Design review of the part built by this model. Coordinates are the model's own, in mm. A direction names the side the tool comes from. Coordinates: 2 decimals unless noted, no trailing zeros. Order: outer loops, then holes, each group sorted by start corner. A loop starts at its lowest first (then second) coordinate and runs counter-clockwise, first axis right, second up. Notation, with made-up numbers: M -33.5,36.5 L 5.5,36.5 A18 ccw 5.5,59.5 Z; hole C -24.5,23 d7. An arc over 180 degrees is marked long. Answer as a JSON object with one key per item and string values.
from build123d import *

# Parameters (mm, degrees)
F0_R     = 16
F0_R_2   = 13.5
F1_DEPTH = 15.5
F2_W     = 4
F2_H     = 19.090906
F3_DEPTH = 25
F4_W     = 2
F4_H     = 0.5
F4_W_2   = 0.5
F4_H_2   = 2
F5_DEPTH = 25


with BuildPart() as f1:
    # F0 (on Front) → F1 (new body)
    with BuildSketch(Plane.XZ):
        Circle(F0_R)
        Circle(F0_R_2, mode=Mode.SUBTRACT)
    extrude(amount=F1_DEPTH)

    # F2 (on Top) → F3 (cut)
    with BuildSketch(Plane.XY):
        with Locations((0, -8.067074)):
            Rectangle(F2_W, F2_H)
    extrude(amount=-F3_DEPTH, mode=Mode.SUBTRACT)

    # F4 (on Front) → F5 (cut, symmetric)
    with BuildSketch(Plane.XZ):
        with Locations((0, 13.665518)):
            Rectangle(F4_W, F4_H)
        Polygon((-5.251188, 12.925427), (-5.09668, 12.449899), (-3.194566, 13.067933), (-3.349075, 13.543461), align=None)
        Polygon((-8.988353, 10.670105), (-8.694461, 10.265597), (-7.076427, 11.441167), (-7.370319, 11.845676), align=None)
        Polygon((-11.845676, 7.370319), (-11.441167, 7.076427), (-10.265597, 8.694461), (-10.670105, 8.988353), align=None)
        Polygon((-13.543461, 3.349075), (-13.067933, 3.194566), (-12.449899, 5.09668), (-12.925427, 5.251188), align=None)
        with Locations((-13.665518, 0)):
            Rectangle(F4_W_2, F4_H_2)
        Polygon((-12.925427, -5.251188), (-12.449899, -5.09668), (-13.067933, -3.194566), (-13.543461, -3.349075), align=None)
        Polygon((-10.670105, -8.988353), (-10.265597, -8.694461), (-11.441167, -7.076427), (-11.845676, -7.370319), align=None)
        Polygon((-7.370319, -11.845676), (-7.076427, -11.441167), (-8.694461, -10.265597), (-8.988353, -10.670105), align=None)
        Polygon((-3.349075, -13.543461), (-3.194566, -13.067933), (-5.09668, -12.449899), (-5.251188, -12.925427), align=None)
        with Locations((0, -13.665518)):
            Rectangle(F4_W, F4_H)
        Polygon((5.251188, -12.925427), (5.09668, -12.449899), (3.194566, -13.067933), (3.349075, -13.543461), align=None)
        Polygon((8.988353, -10.670105), (8.694461, -10.265597), (7.076427, -11.441167), (7.370319, -11.845676), align=None)
        Polygon((11.845676, -7.370319), (11.441167, -7.076427), (10.265597, -8.694461), (10.670105, -8.988353), align=None)
        Polygon((13.543461, -3.349075), (13.067933, -3.194566), (12.449899, -5.09668), (12.925427, -5.251188), align=None)
        with Locations((13.665518, 0)):
            Rectangle(F4_W_2, F4_H_2)
        Polygon((12.925427, 5.251188), (12.449899, 5.09668), (13.067933, 3.194566), (13.543461, 3.349075), align=None)
        Polygon((10.670105, 8.988353), (10.265597, 8.694461), (11.441167, 7.076427), (11.845676, 7.370319), align=None)
        Polygon((7.370319, 11.845676), (7.076427, 11.441167), (8.694461, 10.265597), (8.988353, 10.670105), align=None)
        Polygon((3.349075, 13.543461), (3.194566, 13.067933), (5.09668, 12.449899), (5.251188, 12.925427), align=None)
    extrude(amount=F5_DEPTH, both=True, mode=Mode.SUBTRACT)


solid = f1.part
1) Add section A-A (z = 0). State the section outline as (x, y) points.
Taken from the geometry:
{"outline": "M -16,-15.5 L -13.92,-15.5 L -13.92,0 L -16,0 Z; M 13.92,-15.5 L 16,-15.5 L 16,0 L 13.92,0 Z"}
2) Add section C-C (x = 0). State the section outline as (y, z) points, and give its area (3 significant figures).
Taken from the geometry:
{"outline": "M -15.5,13.92 L 0,13.92 L 0,16 L -15.5,16 Z", "area": "32.3 mm2"}
3) Tool access review of faces 1 (the flat face through (-2, -8, -15)), 2 (the flat face through (-4.31, -7.64, -13.23)): name each direction out of +Z, -Z, +X, -X, +Y, -Y from which nothing blocks a thin tool from reaching the whole face with its end or side.
Taken from the geometry:
{"face 1": "-Z, +Y, -Y", "face 2": "+Y, -Y"}
4) To check wall thickness, follow L1, parallel to X at y = -7.25, z = 0; L2, parallel to X at y = -13, z = -14; L3, parallel to Z at x = 0.5, y = -2.25. State the ranges of each line that lie inside material, in increasing order.
Taken from the geometry:
{"L1": "x = -16 to -13.92, 13.92 to 16", "L2": "x = -7.75 to -2, 2 to 7.75", "L3": "z = 13.92 to 15.99"}
5) Add section B-B (x = -6). State the section outline as (y, z) points.
Taken from the geometry:
{"outline": "M -15.5,-14.83 L 0,-14.83 L 0,-12.09 L -15.5,-12.09 Z; M -15.5,12.09 L 0,12.09 L 0,14.83 L -15.5,14.83 Z"}
6) Insertion check: pin 1 Ø6 at (x, y) = (0, -9) entering from -Z; pin 2 Ø4 at (y, z) = (-5, -2) entering from -X; pin 3 Ø4 at (y, z) = (-12.5, -11.5) entering from +X; pin 4 Ø2 at (y, z) = (-7.5, -14.5) entering from -X. Each pin has a flat end and moves straight along its axis. Give the tip position at first contact, or say it passes through.
Taken from the geometry:
{"pin 1": "stops at z = -15.87", "pin 2": "stops at x = -16", "pin 3": "stops at x = 12.87", "pin 4": "stops at x = -8.59"}
